Here's how the part is built. I have some questions about the finished solid (model axes, mm). A direction names the side the tool comes from. Round coordinates to 2 decimals unless told otherwise and drop trailing zeros. Loops run counter-clockwise (first coordinate to the right, second up) from the corner with the lowest first, then second, coordinate; pieces in that order, holes last. Notation, with made-up numbers: (69.25, 11) -> (82.25, 11) arc R9 ccw to (82.25, 21) -> close; hole circle Ø2 at (6.25, 68.25). An arc over 180 degrees is marked (long way). Use one line per item in the form item = value. Start each with the question number.
Item 1: I'm going to push flat-ended pins straight in: pin 1 Ø8 at (x, z) = (6.5, -6) entering from -Y; pin 2 Ø1.5 at (y, z) = (2.5, 1.5) entering from -X; pin 3 Ø5 at (x, z) = (4.5, -8) entering from -Y. Where does each tip first touch, or does it pass through?
Item 2: If we section it at A-A (y = 0): Write out the boundary of the cut face in (x, z), then the cut area to 3 significant figures.
Item 3: If I drill on L1, parallel to Y at x = 0, z = -10; L2, parallel to Z at x = -5, y = -5; L3, parallel to X at y = -1.75, z = -7, over which ranges is the centre line in solid material (lowest first)? Write a range as [from, to].
Item 4: For faces 1 (the face through (-0.1, -4.3, 10)), 2 (the face through (-0.867, -3.905, -5.21)), 3 (the face through (6.466, -2.681, -14.79)), which set-ups out of +Z, -Z, +X, -X, +Y, -Y let a thin tool reach every point of the face, with its end or its side?
Item 5: Thinking about a two-plate mould opening in Y: for faces 4 (the face through (-2.17, -9.76, 4.93)), 5 (the face through (0, 0, -20)), 6 (the face through (-7, -2, 0)), which applies, released by +Y, released by -Y, zero draft, split by the parting line, or undercut?
Item 6: If we section it at B-B (z = -2.5): Write out the boundary of the cut face in (x, y), then the cut area to 3 significant figures.
Item 7: If we section it at D-D (z = -21): Write out the boundary of the cut face in (x, y).
```python
from build123d import *

# Parameters (mm, degrees)
F0_R     = 7
F0_R_2   = 4
F1_DEPTH = 30
F2_DEPTH = 20
F0_R_3   = 10
F3_DEPTH = 10


with BuildPart() as f1:
    # F0 (on Top) → F1 (new body)
    with BuildSketch(Plane.XY):
        Circle(F0_R)
        Circle(F0_R_2, mode=Mode.SUBTRACT)
        Circle(F0_R_2)
    extrude(amount=-F1_DEPTH)

    # F0 (on Top) → F2 (cut)
    with BuildSketch(Plane.XY):
        Circle(F0_R_2)
    extrude(amount=-F2_DEPTH, mode=Mode.SUBTRACT)

    # F0 (on Top) → F3 (join)
    with BuildSketch(Plane.XY):
        Circle(F0_R_3)
        Circle(F0_R, mode=Mode.SUBTRACT)
        Circle(F0_R)
        Circle(F0_R_2, mode=Mode.SUBTRACT)
    extrude(amount=F3_DEPTH)


solid = f1.part
```
Values found:
q1.pin_1 = -6.54
q1.pin_2 = -9.85
q1.pin_3 = -6.71
q2.outline = (-10, 0) -> (-7, 0) -> (-7, -30) -> (7, -30) -> (7, 0) -> (10, 0) -> (10, 10) -> (4, 10) -> (4, -20) -> (-4, -20) -> (-4, 10) -> (-10, 10) -> close
q2.area = 380 mm2
q3.L1 = [-7, -4], [4, 7]
q3.L2 = [0, 10]
q3.L3 = [-6.78, -3.6], [3.6, 6.78]
q4.face_1 = +Z, +X, -X, +Y, -Y
q4.face_2 = +Z
q4.face_3 = -Z
q5.face_4 = split by the parting line
q5.face_5 = undercut
q5.face_6 = zero draft
q6.outline = circle Ø14 at (0, 0); hole circle Ø8 at (0, 0)
q6.area = 104 mm2
q7.outline = circle Ø14 at (0, 0)
